Geometry: final body of the model. Coordinates: model frame, mm. A direction names the side the tool comes from. Round coordinates to 2 decimals unless told otherwise and drop trailing zeros. Order: outer loops, then holes, each group sorted by start corner. A loop starts at its lowest first (then second) coordinate and runs counter-clockwise, first axis right, second up. Notation, with made-up numbers: M -19,-16 L 31,-16 A10 cw 31,-10 Z; hole C 71.5,-23 d2. An arc over 180 degrees is marked long. Put each result on its own line as item: value. Start each with the question number.
1) Access query for faces 4 (the cylindrical face through (60.14, 10.382, -19.961)), 5 (the cylindrical face through (-1447.318, 19.961, 10.382)), 6 (the flat face through (-1408, -20, 6)). Directions: +Z, -Z, +X, -X, +Y, -Y. A direction counts if a zero-diameter tool reaches every point of the face in a straight line with its end or side. Return the directions, or none.
2) Material intervals for probe 1 along X at (y, z) = (26, -6); probe 2 along Z at (x, y) = (-464, 20); probe 3 along Z at (x, y) = (-1314.5, -4), sorted ascending. Write a range as [from, to].
3) First-contact query: P1, Ø3, axis at x = -241.5, y = 10, coming from the -Z side; P2, Ø1.5, axis at x = -26, z = -23, coming from the +Y side; P3, Ø8, axis at x = -1057.5, y = 11.5, coming from the -Z side. Flat tips, straight axial feed; report the tip coordinate or a pass-through.
4) Section A-A, the plane x = 106.5. Return loops of the section in (y, z).
5) Draft query along X for faces 1 (the cylindrical face through (-694.14, -1.32, -29.97)), 2 (the flat face through (-1588, 0, 0)), 3 (the conical face through (-1462.294, -4.489, -20.213)). Return one class per face: pulls with the +X half, pulls with the -X half, needs draft (parallel to the pull), parting line crosses it, or undercut.
6) Section B-B, the plane x = -1270. Return loops of the section in (y, z), then the cut area to 3 significant figures.
Autodesk Inventor part; units mm, degrees
ref_plane "YZ Plane" through (0, 0, 0) normal (1, 0, 0) x (0, 1, 0)
ref_plane "XZ Plane" through (0, 0, 0) normal (0, 1, 0) x (-1, 0, 0)
ref_plane "XY Plane" through (0, 0, 0) normal (0, 0, 1) x (1, 0, 0)
sketch "Эскиз1" plane through (0, 0, 0) normal (0, 0, 1) x (1, 0, 0)
  line L0 (0, 0) -> (345, 0)
  line L1 (345, 0) -> (345, 20)
  line L2 (345, 20) -> (280, 20)
  line L3 (0, 0) -> (0, 22.5)
  line L4 (0, 22.5) -> (50, 22.5)
  line L5 (50, 22.5) -> (70, 22.5)
  line L6 (250, 22.5) -> (230, 22.5)
  line L7 (250, 22.5) -> (265, 18.9255)
  line L8 (265, 18.9255) -> (280, 20)
  line L9 (82.7171, 19.4628) -> (70, 22.5)
  line L10 (50, 22.5) -> (36.6597, 19.4628)
  line L11 (36.6597, 19.4628) -> (0, 19.4628)
  line L12 (230, 22.5) -> (211.3782, 19.4628)
  line L13 (211.3782, 19.4628) -> (82.7171, 19.4628)
  dimension "d0" = 345
  dimension "d1" = 20
  dimension "d2" = 65
  dimension "d5" = 22.5
  dimension "d6" = 50
  dimension "d7" = 20
  dimension "d8" = 20
  dimension "d15" = 30
revolve "Вращение1" add sketch "Эскиз1" angle 360 about axis through (0, 0, 0) along (1, 0, 0) contours L3 L11 L10 L5 L9 L13 L12 L6 L7 L8 L2 L1 L0
thread "Резьба1"
sketch "Эскиз2" plane through (0, 0, 0) normal (-1, 0, 0) x (0, 0, 1)
  circle A0 centre (0, 0) radius 30
  dimension "d12" = 60
extrude "Выдавливание1" add sketch "Эскиз2" along normal blind 1408
sketch "Эскиз3" plane through (-1408, 0, 0) normal (-1, 0, 0) x (0, 0, 1)
  circle A0 centre (0, 0) radius 22.5
  dimension "d16" = 45
extrude "Выдавливание2" add sketch "Эскиз3" along normal blind 180
sketch "Эскиз4" plane through (0, 0, 0) normal (0, 0, 1) x (1, 0, 0)
  line L0 (-1408, 30) -> (-1408, -30)
  line L1 (-1588, 22.5) -> (-1588, -22.5)
  line L2 (-1408, -22.5) -> (-1408, 22.5)
  line L3 (-1408, 22.5) -> (-1588, 22.5)
  line L4 (-1588, 22.5) -> (-1588, -22.5)
  line L5 (-1656, 0) -> (-1640, 0)
  line L6 (-1541, 22.5) -> (-1633, 22.5)
  line L7 (-1408, 22.5) -> (-1588, 22.5)
  line L8 (-1408, 0) -> (-1408, 20)
  line L9 (-1408, 20) -> (-1432, 20)
  line L10 (-1432, 20) -> (-1434.5, 22.5)
  line L11 (-1408, 22.5) -> (-1588, 22.5)
  line L12 (-1434.5, 22.5) -> (-1460.5, 22.5)
  line L13 (-1408, 22.5) -> (-1588, 22.5)
  line L14 (-1460.5, 22.5) -> (-1463, 20)
  line L15 (-1463, 20) -> (-1488, 20)
  line L16 (-1488, 20) -> (-1490.5, 22.5)
  line L17 (-1408, 22.5) -> (-1588, 22.5)
  line L18 (-1408, 22.5) -> (-1408, 20)
  line L19 (-1490.5, 22.5) -> (-1408, 22.5)
  dimension "d26" = 135
  dimension "d27" = 26
revolve "Вращение2" cut sketch "Эскиз4" angle 360 about axis through (-1656, 0, 0) along (1, 0, 0)
chamfer "Фаска1" distance 2 angle 45 1 edges at (-1588, 0, -22.5)
fillet "Сопряжение1" radius 2 3 edges at (-1488, -20, 0) (-1463, -20, 0) (-1432, -20, 0)
thread "Резьба2"
chamfer "Фаска2" distance 2 angle 45 1 edges at (345, -20, 0)
properties part number "Шток" material "Сталь, углеродистая"
Result sheet:
1. face 4: +X
1. face 5: -X
1. face 6: none
2. probe 1: x = [-1408, 0]
2. probe 2: z = [-22.36, 22.36]
2. probe 3: z = [-29.73, 29.73]
3. P1: stops at z = -28.77
3. P2: stops at y = 20.12
3. P3: stops at z = -29.05
4. outline: C 0,0 d38.93
5. face 1: needs draft
5. face 2: pulls with the -X half
5. face 3: undercut
6. outline: C 0,0 d60
6. area: 2,830 mm2
